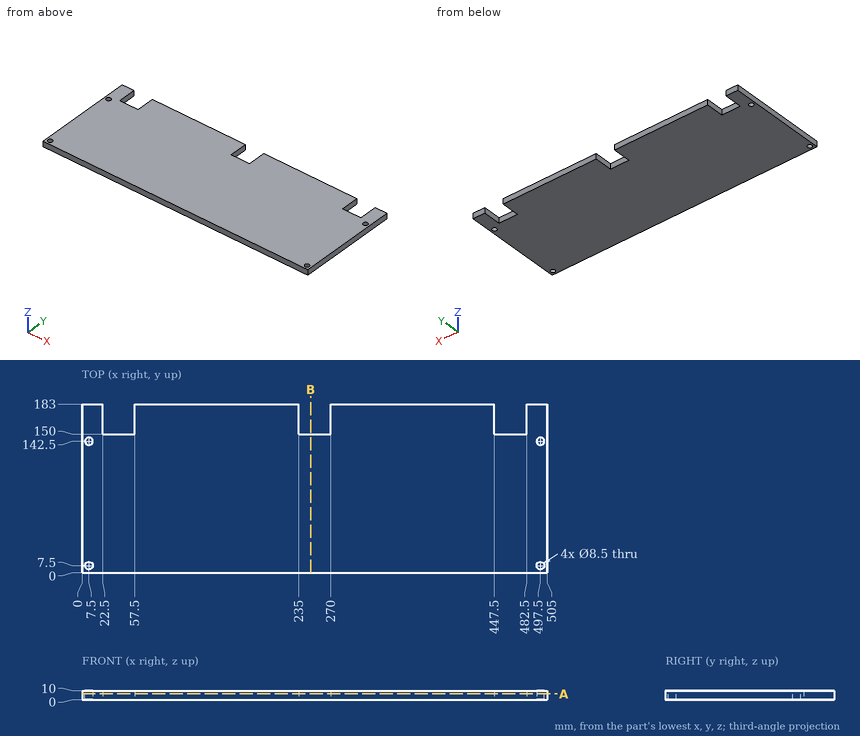
For this review, use the dimensioned drawing (mm, ordinates from the lowest corner) and the shaded views. Round coordinates to 2 decimals unless told otherwise and drop trailing zeros. Order: outer loops, then holes, each group sorted by start corner. A loop starts at its lowest first (then second) coordinate and runs counter-clockwise, first axis right, second up. Notation, with made-up numbers: M 73.5,28 L 109.5,28 A24 ccw 109.5,42 Z; hole C 36.25,11 d8. An arc over 180 degrees is marked long. Write each question's results on one line, items separated by ' | '. Start each with the question number.
1. To check wall thickness, follow L1, parallel to Y at x = 7.5, z = 5; L2, parallel to X at y = 174, z = 7.5; L3, parallel to X at y = 142.5, z = 7.75. State the ranges of each line that lie inside material, in increasing order. Write a range as [from, to].
2. Add section B-B (x = 248). State the section outline as (y, z) points, then the cut area to 3 significant figures.
3. Clearance check with flat-ended pins moving along their axes: pin 1 Ø7 at (x, y) = (497.5, 7.5) entering from -Z; pin 2 Ø3 at (x, z) = (464.5, 6) entering from +Y. State where each tip first meets the part, or that it passes through.
4. Add section A-A (z = 6.5). State the section outline as (x, y) points, then the cut area to 3 significant figures.
Output values:
1) L1: [0, 3.25], [11.75, 138.25], [146.75, 183] | L2: [0, 22.5], [57.5, 235], [270, 447.5], [482.5, 505] | L3: [0, 3.25], [11.75, 493.25], [501.75, 505]
2) outline: M 0,0 L 150,0 L 150,10 L 0,10 Z | area: 1,500 mm^2
3) pin 1: through | pin 2: y = 150
4) outline: M 0,0 L 505,0 L 505,183 L 482.5,183 L 482.5,150 L 447.5,150 L 447.5,183 L 270,183 L 270,150 L 235,150 L 235,183 L 57.5,183 L 57.5,150 L 22.5,150 L 22.5,183 L 0,183 Z; hole C 7.5,7.5 d8.5; hole C 7.5,142.5 d8.5; hole C 497.5,7.5 d8.5; hole C 497.5,142.5 d8.5 | area: 88,700 mm^2
